Could you check a few things on this model? Use its own coordinates, in mm. Give positions to 0.01 mm unless a question says otherwise; leave off trailing zeros. Loops run counter-clockwise (first coordinate to the right, second up) from the corner with the lowest first, then second, coordinate; pieces in that order, holes last. Notation, with made-up numbers: (45, -0.75) -> (96, -0.75) arc R17 ccw to (96, 22.25) -> close; hole circle Ø5 at (40, 72). An arc over 180 degrees is marked (long way). Write item = value, one per line. Start each with the question number.
1) I want a section at A-A (y = 2). List the corners of the cut face in (x, z) for me.
2) I need wall thicknesses on probe 1 along X at (y, z) = (1.1, -80); probe 2 along Z at (x, y) = (-22, 1.35); probe 3 along Z at (x, y) = (15.5, 1.85). Which ranges of each line are inside material? Lowest first, please. Write a range as from..to.
3) I want a section at D-D (x = 8.5). List the corners of the cut face in (y, z) for me.
4) I want a section at B-B (x = -4). List the corners of the cut face in (y, z) for me.
5) I want a section at C-C (z = -80). List the corners of the cut face in (x, y) for me.
6) I'm going to push flat-ended pins straight in: pin 1 Ø1 at (y, z) = (3.5, -4) entering from -X; pin 2 Ø3.5 at (x, z) = (43.71, -58.79) entering from +Y; pin 3 Ø1.5 at (x, y) = (-40.5, 2) entering from +Z; pin 4 Ø1.5 at (y, z) = (2, -15) entering from +X. Where does each tip first touch, or does it pass through?
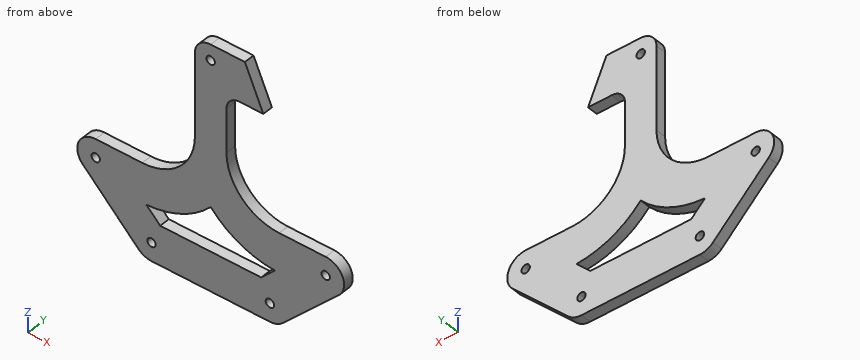
from build123d import *

# Parameters (mm, degrees)
SKETCH1_R           = 3
SKETCH1_R_2         = 1.6
BOSS_EXTRUDE1_DEPTH = 4


with BuildPart() as part:
    # Sketch1 → Boss-Extrude1 (new body)
    with BuildSketch(Plane(origin=(0, 0, 0), x_dir=(1, 0, 0), z_dir=(0, 1, 0))):
        with BuildLine():
            Line((11, 10), (20, 10))
            Line((20, 10), (13, -6))
            Line((13, -6), (0, -6))
            ThreePointArc((0, -6), (-4.242640687, -4.242640687), (-6, 0))
            Line((-6, 0), (-6, 31.786796564))
            ThreePointArc((-6, 31.786796564), (-11.857864376, 45.928932188), (-26, 51.786796564))
            Line((-26, 51.786796564), (-43.713203436, 51.786796564))
            ThreePointArc((-43.713203436, 51.786796564), (-50.180360163, 56.108012538), (-48.662950904, 63.736544033))
            Line((-48.662950904, 63.736544033), (-27.449747468, 84.949747468))
            ThreePointArc((-27.449747468, 84.949747468), (-25.178784027, 86.467156728), (-22.5, 87))
            Line((-22.5, 87), (22.5, 87))
            ThreePointArc((22.5, 87), (25.178784027, 86.467156728), (27.449747468, 84.949747468))
            Line((27.449747468, 84.949747468), (48.662950904, 63.736544033))
            ThreePointArc((48.662950904, 63.736544033), (50.180360163, 56.108012538), (43.713203436, 51.786796564))
            Line((43.713203436, 51.786796564), (26, 51.786796564))
            ThreePointArc((26, 51.786796564), (11.857864376, 45.928932188), (6, 31.786796564))
            Line((6, 31.786796564), (6, 15))
            ThreePointArc((6, 15), (7.464466094, 11.464466094), (11, 10))
        make_face()
        with Locations((-22.5, 80)):
            Circle(SKETCH1_R, mode=Mode.SUBTRACT)
        with Locations((22.5, 80)):
            Circle(SKETCH1_R, mode=Mode.SUBTRACT)
        Circle(SKETCH1_R, mode=Mode.SUBTRACT)
        with Locations((-43.713203436, 58.786796564)):
            Circle(SKETCH1_R, mode=Mode.SUBTRACT)
        with Locations((43.713203436, 58.786796564)):
            Circle(SKETCH1_R, mode=Mode.SUBTRACT)
        with BuildLine():
            ThreePointArc((24.434522737, 66.751768764), (11.059335348, 63.437650262), (0, 55.217545592))
            ThreePointArc((0, 55.217545592), (-11.059335348, 63.437650262), (-24.434522737, 66.751768764))
            Line((-24.434522737, 66.751768764), (-19.186291501, 72))
            Line((-19.186291501, 72), (19.186291501, 72))
            Line((19.186291501, 72), (24.434522737, 66.751768764))
        make_face(mode=Mode.SUBTRACT)
        Circle(SKETCH1_R)
        with Locations(Location((0, 0, 0), (0, 0, 270))):
            Circle(SKETCH1_R_2, mode=Mode.SUBTRACT)
        with Locations((43.713203436, 58.786796564)):
            Circle(SKETCH1_R)
        with Locations(Location((43.713203436, 58.786796564, 0), (0, 0, 270))):
            Circle(SKETCH1_R_2, mode=Mode.SUBTRACT)
        with Locations((22.5, 80)):
            Circle(SKETCH1_R)
        with Locations(Location((22.5, 80, 0), (0, 0, 270))):
            Circle(SKETCH1_R_2, mode=Mode.SUBTRACT)
        with Locations((-22.5, 80)):
            Circle(SKETCH1_R)
        with Locations(Location((-22.5, 80, 0), (0, 0, 270))):
            Circle(SKETCH1_R_2, mode=Mode.SUBTRACT)
        with Locations((-43.713203436, 58.786796564)):
            Circle(SKETCH1_R)
        with Locations(Location((-43.713203436, 58.786796564, 0), (0, 0, 270))):
            Circle(SKETCH1_R_2, mode=Mode.SUBTRACT)
    extrude(amount=BOSS_EXTRUDE1_DEPTH)


solid = part.part
Answer list:
q1.outline = (-48.66, -63.74) -> (-27.45, -84.95) arc R7 ccw to (-22.5, -87) -> (22.5, -87) arc R7 ccw to (27.45, -84.95) -> (48.66, -63.74) arc R7 ccw to (43.71, -51.79) -> (26, -51.79) arc R20 cw to (6, -31.79) -> (6, -15) arc R5 cw to (11, -10) -> (20, -10) -> (13, 6) -> (0, 6) arc R6 ccw to (-6, 0) -> (-6, -31.79) arc R20 cw to (-26, -51.79) -> (-43.71, -51.79) arc R7 ccw to start; hole circle Ø3.2 at (-43.71, -58.79); hole (-24.43, -66.75) -> (-19.19, -72) -> (19.19, -72) -> (24.43, -66.75) arc R35 cw to (0, -55.22) arc R35 cw to start; hole circle Ø3.2 at (-22.5, -80); hole circle Ø3.2 at (0, 0); hole circle Ø3.2 at (22.5, -80); hole circle Ø3.2 at (43.71, -58.79)
q2.probe_1 = -32.4..-24.1, -20.9..20.9, 24.1..32.4
q2.probe_2 = -87..-81.52, -78.48..-69.19, -66.56..-51.38
q2.probe_3 = -87..-72, -65.17..-48.81, -10..0.29
q3.outline = (0, -87) -> (4, -87) -> (4, -72) -> (0, -72) -> close; (0, -62.1) -> (4, -62.1) -> (4, -41.47) -> (0, -41.47) -> close; (0, -10.67) -> (4, -10.67) -> (4, 6) -> (0, 6) -> close
q4.outline = (0, -87) -> (4, -87) -> (4, -72) -> (0, -72) -> close; (0, -59.01) -> (4, -59.01) -> (4, 4.47) -> (0, 4.47) -> close
q5.outline = (-32.4, 0) -> (-24.1, 0) -> (-24.1, 4) -> (-32.4, 4) -> close; (-20.9, 0) -> (20.9, 0) -> (20.9, 4) -> (-20.9, 4) -> close; (24.1, 0) -> (32.4, 0) -> (32.4, 4) -> (24.1, 4) -> close
q6.pin_1 = -6
q6.pin_2 = 4
q6.pin_3 = -51.79
q6.pin_4 = 6.06
